Can you work these out from the drawing? Everything is in mm from the part's minimum corner. Round coordinates to 2 decimals unless told otherwise and drop trailing zeros. Loops run counter-clockwise (first coordinate to the right, second up) from the corner with the lowest first, then second, coordinate; pieces in that order, holes last. Notation, with made-up numbers: M -6.75,51.5 L 21.25,51.5 A20 ccw 21.25,80.5 Z; hole C 38.5,22.5 d4. An arc over 180 degrees is marked long. Use a Markdown table: item, result.
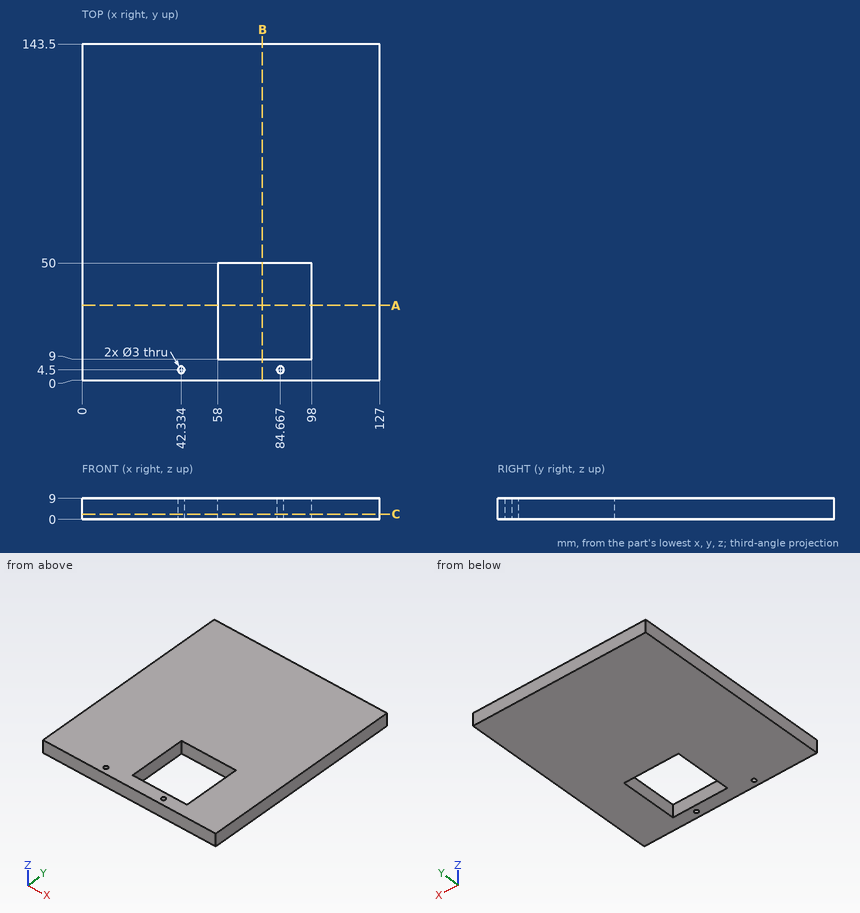
Q1. Imagine slicing it at B-B, the plane x = 77. Please give me the cut outline in (y, z).
Return value:
| item | result |
|---|---|
| outline | M 0,0 L 9,0 L 9,9 L 0,9 Z; M 50,0 L 143.5,0 L 143.5,9 L 50,9 Z |
Q2. Imagine slicing it at A-A, the plane y = 32. Please give me the cut outline in (x, z).
Return value:
| item | result |
|---|---|
| outline | M 0,0 L 58,0 L 58,9 L 0,9 Z; M 98,0 L 127,0 L 127,9 L 98,9 Z |
Q3. Will this pin go through, and if not, where does the flat tip stop? P1, Ø5, axis at y = 46, z = 1, coming from the -X side.
Return value:
| item | result |
|---|---|
| P1 | stops at x = 0 |
Q4. I need wall thicknesses on line 1 (X direction, y = 46.5, z = 1.75); line 2 (Y direction, x = 77.5, z = 5.25). Which ranges of each line are inside material? Lowest first, please. Write a range as from..to.
Return value:
| item | result |
|---|---|
| line 1 | x = 0..58, 98..127 |
| line 2 | y = 0..9, 50..143.5 |
Q5. Imagine slicing it at C-C, the plane z = 2.25. Please give me the cut outline in (x, y), then the cut area to 3 significant figures.
Return value:
| item | result |
|---|---|
| outline | M 0,0 L 127,0 L 127,143.5 L 0,143.5 Z; hole C 42.33,4.5 d3; hole M 58,9 L 98,9 L 98,50 L 58,50 Z; hole C 84.67,4.5 d3 |
| area | 16,600 mm^2 |
